Autodesk Inventor part; units mm, degrees
ref_plane "YZ Plane" through (0, 0, 0) normal (1, 0, 0) x (0, 1, 0)
ref_plane "XZ Plane" through (0, 0, 0) normal (0, 1, 0) x (-1, 0, 0)
ref_plane "XY Plane" through (0, 0, 0) normal (0, 0, 1) x (1, 0, 0)
sketch "Эскиз1" plane through (0, 0, 0) normal (0, 1, 0) x (-1, 0, 0)
  arc A0 (313.5, 70) -> (307.5, 64) centre (313.5, 64) ccw
  line L0 (307.5, 0) -> (307.5, 64)
  line L1 (320, 0) -> (307.5, 0)
  line L2 (320, 70) -> (320, 0)
  line L3 (313.5, 70) -> (320, 70)
  arc A1 (307.5, 126) -> (313.5, 120) centre (313.5, 126) ccw
  line L4 (320, 120) -> (313.5, 120)
  line L5 (320, 190) -> (320, 120)
  line L6 (307.5, 190) -> (320, 190)
  line L7 (307.5, 126) -> (307.5, 190)
  arc A2 (6.5, 120) -> (12.5, 126) centre (6.5, 126) ccw
  line L8 (12.5, 190) -> (12.5, 126)
  line L9 (0, 190) -> (12.5, 190)
  line L10 (0, 120) -> (0, 190)
  line L11 (6.5, 120) -> (0, 120)
  line L12 (12.5, 64) -> (12.5, 0)
  arc A3 (12.5, 64) -> (6.5, 70) centre (6.5, 64) ccw
  line L13 (0, 70) -> (6.5, 70)
  line L14 (0, 0) -> (0, 70)
  line L15 (12.5, 0) -> (0, 0)
  line L16 (12.5, 64) -> (12.5, 0)
  point P0 (144, 0)
extrude "Выдавливание1" add sketch "Эскиз1" along normal blind 15
sketch "Эскиз2" plane through (0, 15, 0) normal (0, 1, 0) x (1, 0, 0)
  line L0 (-320, -120) -> (-320, -190)
  line L1 (-320, -190) -> (-295, -190)
  line L2 (-295, -190) -> (-295, 0)
  line L3 (-295, 0) -> (-320, 0)
  line L4 (-320, 0) -> (-320, -190)
  line L5 (0, -190) -> (0, -120)
  line L6 (0, -190) -> (-25, -190)
  line L7 (-25, -190) -> (-25, 0)
  line L8 (-25, 0) -> (0, 0)
  line L9 (0, 0) -> (0, -190)
  point P0 (0, 0)
  dimension "d2" = 25
  dimension "d3" = 25
extrude "Выдавливание2" add sketch "Эскиз2" along normal blind 60
sketch "Эскиз3" plane through (0, 75, 0) normal (0, 1, 0) x (1, 0, 0)
  line L0 (-320, 0) -> (-320, -190)
  line L1 (-320, -190) -> (81, -190)
  line L2 (81, -190) -> (81, 0)
  line L3 (81, 0) -> (-320, 0)
  line L4 (-320, 0) -> (-320, -190)
  point P0 (0, 0)
extrude "Выдавливание3" add sketch "Эскиз3" along normal blind 20
properties part number "BackPlate"
CAD build for the part. Positions are in the model's coordinates, mm. A direction names the side the tool comes from. Give positions to 0.01 mm unless a question says otherwise; leave off trailing zeros. Loops run counter-clockwise (first coordinate to the right, second up) from the corner with the lowest first, then second, coordinate; pieces in that order, holes last. Notation, with made-up numbers: (69.25, -34.5) - (106.25, -34.5) arc R13 ccw to (106.25, -12.5) - close; hole circle Ø10 at (-14.75, -17). An arc over 180 degrees is marked (long way). Put each result on its own line as item: value.
Q1. Probe line 1 along X through (y, z) = (69.5, 19); line 2 along Y through (x, z) = (-92, 107); line 3 along Y through (x, z) = (-296, 25.5). List the from-to ranges inside material, lowest first.
Filled in:
line 1: x = -320 to -295, -25 to 0
line 2: y = 75 to 95
line 3: y = 15 to 95
Q2. Slice it at D-D (x = -182). Give the cut face in (y, z), plus the area to 3 significant figures.
Filled in:
outline: (75, 0) - (95, 0) - (95, 190) - (75, 190) - close
area: 3,800 mm²
Q3. Tool access for faces 1 (the face through (0, 37, 94)), 2 (the face through (-6, 0, 155)), 3 (the face through (-12.5, 7, 32)): list every direction of +Z, -Z, +X, -X, +Y, -Y with a clear straight run to the whole face (end or side of a thin tool).
Filled in:
face 1: +Z, -Z, +X, -Y
face 2: +Z, -Z, +X, -X, -Y
face 3: +Z, -Z, -Y
Q4. Flat gauge pin, fed straight in: pin 1 (16.5 mm diameter, centred on y = 4, z = 45.5, fed in from +X). Where does the tip first touch, or does it go through?
Filled in:
pin 1: stops at x = 0
Q5. Slice it at A-A (y = 8). Give the cut face in (x, z).
Filled in:
outline: (-320, 0) - (-307.5, 0) - (-307.5, 64) arc R6 ccw to (-313.5, 70) - (-320, 70) - close; (-320, 120) - (-313.5, 120) arc R6 ccw to (-307.5, 126) - (-307.5, 190) - (-320, 190) - close; (-12.5, 0) - (0, 0) - (0, 70) - (-6.5, 70) arc R6 ccw to (-12.5, 64) - close; (-12.5, 126) arc R6 ccw to (-6.5, 120) - (0, 120) - (0, 190) - (-12.5, 190) - close
Q6. Slice it at B-B (z = 161.5). Give the cut face in (x, y).
Filled in:
outline: (-320, 0) - (-307.5, 0) - (-307.5, 15) - (-295, 15) - (-295, 75) - (-25, 75) - (-25, 15) - (-12.5, 15) - (-12.5, 0) - (0, 0) - (0, 75) - (81, 75) - (81, 95) - (-320, 95) - close
Q7. Slice it at C-C (y = 66). Give the cut face in (x, z), plus the area to 3 significant figures.
Filled in:
outline: (-320, 0) - (-295, 0) - (-295, 190) - (-320, 190) - close; (-25, 0) - (0, 0) - (0, 190) - (-25, 190) - close
area: 9,500 mm²
Q8. Mould opens along Z. For faces 4 (the face through (-307.5, 7, 32)), 5 (the face through (-15, 15, 94)), 6 (the face through (-135, 79, 190)), 7 (the face through (-305, 15, 94)) say: pulls with the +Z half, pulls with the -Z half, needs draft (parallel to the pull), parting line crosses it, or undercut.
Filled in:
face 4: needs draft
face 5: undercut
face 6: pulls with the +Z half
face 7: undercut
